from build123d import *

# Parameters (mm, degrees)
BASE_FLANGE1_DEPTH           = 3.2639
F_10_0_1935_DIAMETER_HOLE1_D = 4.9149
FILLET1_R                    = 1.5875
FILLET2_R                    = 12.7
FILLET3_R                    = 25.4


# Sheet-metal steps are written as plain solids
with BuildPart() as part:
    # Sketch1 → Base-Flange1 (new body)
    with BuildSketch(Plane.XY):
        with BuildLine():
            Line((-175.064802987, -46.731119967), (-166.42876849, -39.737797122))
            Line((-166.42876849, -39.737797122), (-177.418275819, -26.16688577))
            Line((-177.418275819, -26.16688577), (-186.054310315, -33.160208616))
            Line((-186.054310315, -33.160208616), (-203.965209169, -11.04209055))
            Line((-203.965209169, -11.04209055), (-303.890728914, -91.960180949))
            ThreePointArc((-303.890728914, -91.960180949), (0, -317.5), (303.890728914, -91.960180949))
            Line((303.890728914, -91.960180949), (203.965209169, -11.04209055))
            Line((203.965209169, -11.04209055), (186.054310315, -33.160208616))
            Line((186.054310315, -33.160208616), (177.418275819, -26.16688577))
            Line((177.418275819, -26.16688577), (166.42876849, -39.737797122))
            Line((166.42876849, -39.737797122), (175.064802987, -46.731119967))
            Line((175.064802987, -46.731119967), (157.153904133, -68.849238033))
            Line((157.153904133, -68.849238033), (38.1, -164.30625))
            Line((38.1, -164.30625), (8.73125, -164.30625))
            Line((8.73125, -164.30625), (8.73125, -153.19375))
            Line((8.73125, -153.19375), (-8.73125, -153.19375))
            Line((-8.73125, -153.19375), (-8.73125, -164.30625))
            Line((-8.73125, -164.30625), (-38.1, -164.30625))
            Line((-38.1, -164.30625), (-157.153904133, -68.849238033))
            Line((-157.153904133, -68.849238033), (-175.064802987, -46.731119967))
        make_face()
        with BuildLine():
            ThreePointArc((-175.925266574, -225.174072843), (-142.875, -247.466759131), (-107.043834069, -264.942786442))
            ThreePointArc((-107.043834069, -264.942786442), (-49.179248656, -240.380727184), (-73.741307914, -182.516141771))
            ThreePointArc((-73.741307914, -182.516141771), (-98.425, -170.477100735), (-121.192961418, -155.119916847))
            ThreePointArc((-121.192961418, -155.119916847), (-183.586191994, -162.780842267), (-175.925266574, -225.174072843))
        make_face(mode=Mode.SUBTRACT)
        with BuildLine():
            ThreePointArc((175.925266574, -225.174072843), (142.875, -247.466759131), (107.043834069, -264.942786442))
            ThreePointArc((107.043834069, -264.942786442), (49.179248656, -240.380727184), (73.741307914, -182.516141771))
            ThreePointArc((73.741307914, -182.516141771), (98.425, -170.477100735), (121.192961418, -155.119916847))
            ThreePointArc((121.192961418, -155.119916847), (183.586191994, -162.780842267), (175.925266574, -225.174072843))
        make_face(mode=Mode.SUBTRACT)
    extrude(amount=-BASE_FLANGE1_DEPTH)

    # #10 (0.1935) Diameter Hole1 (through all)
    with Locations(Plane.XY):
        with Locations((-200.299064072, -55.930402224), (-264.45246319, -107.880800505), (0, -189.70625), (0, -284.95625), (200.299064072, -55.930402224), (264.45246319, -107.880800505)):
            Hole(F_10_0_1935_DIAMETER_HOLE1_D / 2)

    # Fillet1
    fillet1_edges = [part.edges().sort_by_distance(p)[0] for p in [
        (-8.73125, -164.30625, -1.63195),
        (-8.73125, -153.19375, -1.63195),
        (8.73125, -153.19375, -1.63195),
        (8.73125, -164.30625, -1.63195),
        (175.064802987, -46.731119967, -1.63195),
        (166.42876849, -39.737797122, -1.63195),
        (177.418275819, -26.16688577, -1.63195),
        (186.054310315, -33.160208616, -1.63195),
        (-186.054310315, -33.160208616, -1.63195),
        (-177.418275819, -26.16688577, -1.63195),
        (-166.42876849, -39.737797122, -1.63195),
        (-175.064802987, -46.731119967, -1.63195),
    ]]
    fillet(fillet1_edges, radius=FILLET1_R)

    # Fillet2
    fillet2_edges = [part.edges().sort_by_distance(p)[0] for p in [
        (-38.1, -164.30625, -1.63195),
        (38.1, -164.30625, -1.63195),
        (157.153904133, -68.849238033, -1.63195),
        (203.965209169, -11.04209055, -1.63195),
        (-203.965209169, -11.04209055, -1.63195),
        (-157.153904133, -68.849238033, -1.63195),
    ]]
    fillet(fillet2_edges, radius=FILLET2_R)

    # Fillet3
    fillet3_edges = [part.edges().sort_by_distance(p)[0] for p in [
        (303.890728914, -91.960180949, -1.63195),
        (-303.890728914, -91.960180949, -1.63195),
    ]]
    fillet(fillet3_edges, radius=FILLET3_R)


solid = part.part
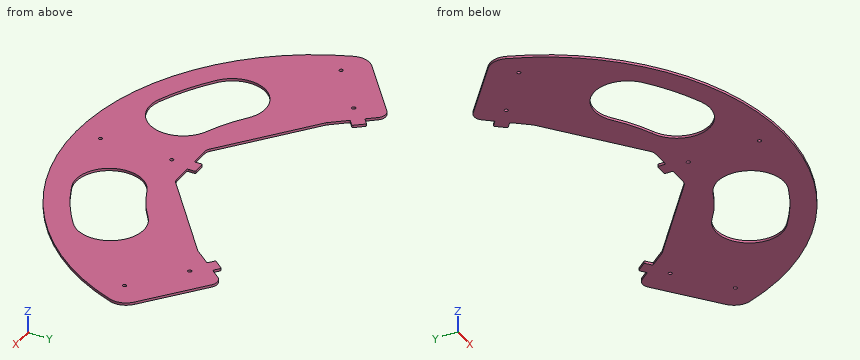
Here's how the part is built. I have some questions about the finished solid (model axes, mm). Give positions to 0.01 mm unless a question says otherwise; leave off trailing zeros. Order: outer loops, then holes, each group sorted by start corner. A loop starts at its lowest first (then second) coordinate and runs counter-clockwise, first axis right, second up. Notation, with made-up numbers: (48, -35.75) -> (67, -35.75) arc R23 ccw to (67, -9.75) -> close; hole circle Ø11 at (22, -28.75). An arc over 180 degrees is marked (long way). One line per item, written item: value. Start each with the question number.
1. Imagine slicing it at B-B, the plane x = 67. List the corners of the cut face in (y, z) for me, plus the area to 3 significant figures.
2. Imagine slicing it at C-C, the plane y = -95. List the corners of the cut face in (x, z) for me.
3. Imagine slicing it at A-A, the plane y = -240.5. List the corners of the cut face in (x, z) for me, plus the area to 3 significant figures.
4. I need wall thicknesses on probe 1 along X at (y, z) = (-191.5, -1.7); probe 2 along X at (y, z) = (-106.5, -1.55); probe 3 along Y at (x, z) = (-5.5, -0.65). Which ranges of each line are inside material? Lowest first, please. Write a range as from..to.
5. Imagine slicing it at D-D, the plane z = -2.15. Count the separate pieces of the cut face and the enclosed holes in it, plus the area to 3 significant figures.
Values follow:
1. outline: (-310.35, -3.26) -> (-261.53, -3.26) -> (-261.53, 0) -> (-310.35, 0) -> close; (-185.93, -3.26) -> (-141.13, -3.26) -> (-141.13, 0) -> (-185.93, 0) -> close
1. area: 306 mm2
2. outline: (-298.99, -3.26) -> (-124.54, -3.26) -> (-124.54, 0) -> (-298.99, 0) -> close; (124.54, -3.26) -> (298.99, -3.26) -> (298.99, 0) -> (124.54, 0) -> close
3. outline: (-207.28, -3.26) -> (-154.31, -3.26) -> (-154.31, 0) -> (-207.28, 0) -> close; (-49.23, -3.26) -> (49.23, -3.26) -> (49.23, 0) -> (-49.23, 0) -> close; (154.31, -3.26) -> (207.28, -3.26) -> (207.28, 0) -> (154.31, 0) -> close
3. area: 667 mm2
4. probe 1: x = -253.25..-192.99, -59.78..-1.68, 1.68..59.78, 192.99..253.25
4. probe 2: x = -298.93..-266.49, -262.42..-110.2, 110.2..262.42, 266.49..298.93
4. probe 3: y = -317.45..-153.19
5. separate pieces: 1
5. enclosed holes: 8
5. area: 78,300 mm2
